Verification items for the finished model (mm, model axes). A direction names the side the tool comes from. Coordinates: 2 decimals unless noted, no trailing zeros. Order: outer loops, then holes, each group sorted by start corner. A loop starts at its lowest first (then second) coordinate and runs counter-clockwise, first axis right, second up. Notation, with made-up numbers: (54, -35.5) -> (104, -35.5) arc R26 ccw to (104, 3.5) -> close; hole circle Ø3 at (27, -36). An arc over 180 degrees is marked (long way). Use CSV: the item, a comma, the result in double quotes. Start each with the question number.
1) Release check for a two-part mould opening along Z. For faces 4 (the cylindrical face through (-1.08, 1.24, -4.88)), 5 (the flat face through (0, 8, -7)), 6 (the cylindrical face through (7.62, 5.7, 3.16)) record: released by +Z, released by -Z, zero draft, split by the parting line, or undercut.
2) Sectioned sample at C-C on y = 4.5. Record the boundary of the cut face in (x, z).
3) Sectioned sample at A-A on z = 0. Record the boundary of the cut face in (x, y), then the cut area to 3 significant figures.
4) Sectioned sample at B-B on x = 0. Record the boundary of the cut face in (y, z), then the cut area to 3 significant figures.
5) Scan lines: line 1 along Z through (x, y) = (0, 4.9); line 2 along Z through (x, y) = (0, 1.4); line 3 along Y through (x, z) = (6, 1.75). Record each from-to range of solid material in increasing order.
6) Tool access check on faces 1 (the flat face through (5, 2, -2)), 2 (the cylindrical face through (-1.38, 5.73, -6.2)), 3 (the flat face through (-4, 0, -4)). Record the directions out of +Z, -Z, +X, -X, +Y, -Y that give a thin tool (end or side, any length) a straight path to the whole face; none if there is none.
7) Go/stop test with flat-tipped pins: pin 1 (3 mm diameter, centred on y = 6, z = 0, fed in from +X); pin 2 (1 mm diameter, centred on x = -2.5, z = -6.5, fed in from -Y); pin 3 (4.5 mm diameter, centred on x = -2, z = 2, fed in from +Y); pin 4 (1.5 mm diameter, centred on x = 2.5, z = -1, fed in from -Y). Record where each tip stops, or that it passes through.
Autodesk Inventor part; units mm, degrees
ref_plane "YZ Plane" through (0, 0, 0) normal (1, 0, 0) x (0, 1, 0)
ref_plane "XZ Plane" through (0, 0, 0) normal (0, 1, 0) x (-1, 0, 0)
ref_plane "XY Plane" through (0, 0, 0) normal (0, 0, 1) x (1, 0, 0)
sketch "Sketch1" plane through (0, 0, 0) normal (0, 0, 1) x (1, 0, 0)
  line L0 (0, 10.7366) -> (0, -7.1166)
  line L1 (0, 0) -> (9.5, 0)
  line L2 (9.5, 0) -> (9.5, 2)
  line L3 (9.5, 2) -> (8.25, 2)
  line L4 (8.25, 2) -> (8.25, 8)
  line L5 (8.25, 8) -> (6.35, 8)
  line L6 (6.35, 8) -> (6.35, 2)
  line L7 (6.35, 2) -> (0, 2)
  dimension "d0" = 19
  dimension "d1" = 12.7
  dimension "d2" = 1.9
  dimension "d3" = 2
  dimension "d6" = 6
revolve "Revolution1" add sketch "Sketch1" angle 360 about axis through (0, 10.7366, 0) along (0, -1, 0)
sketch "Sketch2" plane through (0, 0, 0) normal (0, 0, 1) x (1, 0, 0)
  line L0 (6.1122, 2) -> (7.35, 2)
  line L1 (8.25, 8) -> (8.25, 2)
  line L2 (7.35, 4) -> (6.1122, 4)
  line L3 (6.1122, 4) -> (6.1122, 2)
  line L4 (8.25, 3) -> (8.25, 4)
  line L5 (-8.25, 8) -> (8.25, 8)
  line L6 (0, 5.3477) -> (0, 2.8187)
  line L7 (7.35, 4) -> (7.35, 2)
  point P0 (0, 0)
  dimension "d7" = 4
  dimension "d8" = 2
  dimension "d9" = 14.7
revolve "Revolution2" cut sketch "Sketch2" angle 360 about axis through (0, 5.3477, 0) along (0, -1, 0)
sketch "Sketch3" plane through (0, 0, 0) normal (0, -1, 0) x (1, 0, 0)
  circle A0 centre (0, 0) radius 5
  dimension "d11" = 10
extrude "Extrusion1" cut sketch "Sketch3" against normal up to surface (2 mm away)
fillet "Fillet1" radius 2 1 edges at (-8.25, 2, 0)
fillet "Fillet2" radius 0.5 2 edges at (-6.35, 8, 0) (-8.25, 8, 0)
fillet "Fillet3" radius 0.5 2 edges at (-9.5, 0, 0) (-5, 0, 0)
properties part number "çıkçıkkarşılıkk"
Answers follow:
1,face 4,"undercut"
1,face 5,"zero draft"
1,face 6,"split by the parting line"
2,outline,"circle Ø16.5 at (0, 0); hole circle Ø12.7 at (0, 0)"
3,outline,"(-9.5, 0.5) arc R0.5 ccw to (-9, 0) -> (-5.5, 0) arc R0.5 ccw to (-5, 0.5) -> (-5, 2) -> (-7.35, 2) -> (-7.35, 4) -> (-6.35, 4) -> (-6.35, 7.5) arc R0.5 ccw to (-6.85, 8) -> (-7.75, 8) arc R0.5 ccw to (-8.25, 7.5) -> (-8.25, 3.85) arc R2 cw to (-9.5, 2) -> close; (5, 0.5) arc R0.5 ccw to (5.5, 0) -> (9, 0) arc R0.5 ccw to (9.5, 0.5) -> (9.5, 2) arc R2 cw to (8.25, 3.85) -> (8.25, 7.5) arc R0.5 ccw to (7.75, 8) -> (6.85, 8) arc R0.5 ccw to (6.35, 7.5) -> (6.35, 4) -> (7.35, 4) -> (7.35, 2) -> (5, 2) -> close"
3,area,"37.7 mm²"
4,outline,"(0, -9) arc R0.5 ccw to (0.5, -9.5) -> (2, -9.5) arc R2 cw to (3.85, -8.25) -> (7.5, -8.25) arc R0.5 ccw to (8, -7.75) -> (8, -6.85) arc R0.5 ccw to (7.5, -6.35) -> (4, -6.35) -> (4, -7.35) -> (2, -7.35) -> (2, -5) -> (0.5, -5) arc R0.5 ccw to (0, -5.5) -> close; (0, 5.5) arc R0.5 ccw to (0.5, 5) -> (2, 5) -> (2, 7.35) -> (4, 7.35) -> (4, 6.35) -> (7.5, 6.35) arc R0.5 ccw to (8, 6.85) -> (8, 7.75) arc R0.5 ccw to (7.5, 8.25) -> (3.85, 8.25) arc R2 cw to (2, 9.5) -> (0.5, 9.5) arc R0.5 ccw to (0, 9) -> close"
4,area,"37.7 mm²"
5,line 1,"z = -8.25 to -6.35, 6.35 to 8.25"
5,line 2,"z = -9.5 to -5, 5 to 9.5"
5,line 3,"y = 0 to 2"
6,face 1,"none"
6,face 2,"+Y"
6,face 3,"+Z, -Z, +X, -X, -Y"
7,pin 1,"stops at x = 8.25"
7,pin 2,"stops at y = 0"
7,pin 3,"stops at y = 2"
7,pin 4,"passes through"
